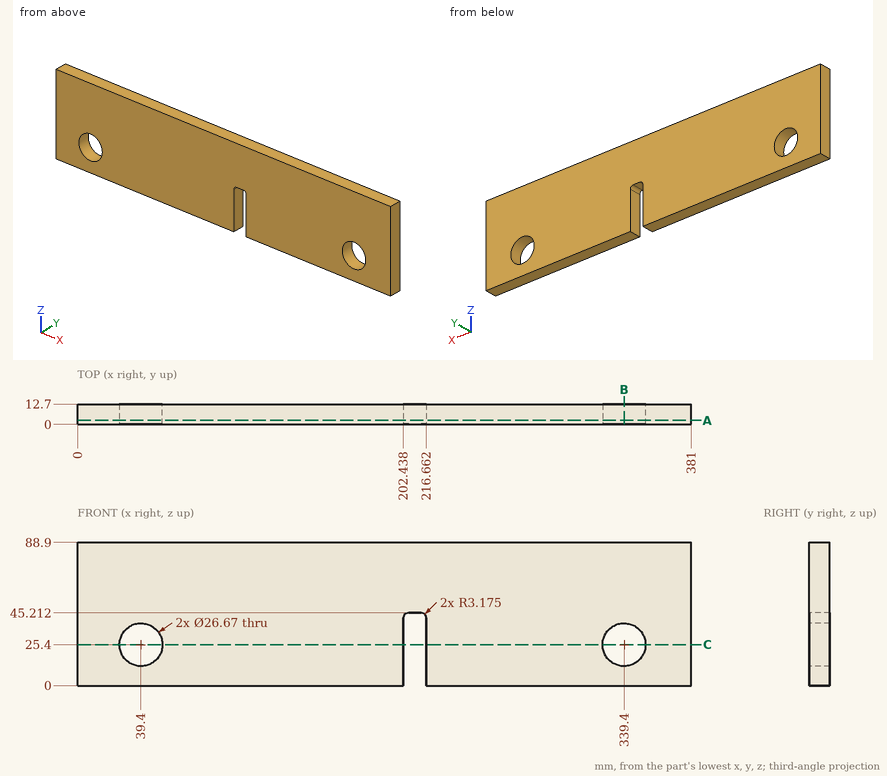
The drawing under review shows one solid part. Ordinate dimensions are in mm from its lowest x, y, z. Round coordinates to 2 decimals unless told otherwise and drop trailing zeros. Loops run counter-clockwise (first coordinate to the right, second up) from the corner with the lowest first, then second, coordinate; pieces in that order, holes last. Notation, with made-up numbers: (13, 89.25) -> (40, 89.25) arc R27 cw to (40, 108.25) -> close; hole circle Ø7 at (22, 71.25). An arc over 180 degrees is marked (long way). One line per question, with ' | ' between items. Start each with the question number.
Item 1: Add section B-B, the plane x = 339.4. Write out the cut boundary in (y, z) (3 decimals), then the cut area to 3 significant figures.
Item 2: Wall thickness on line 1 along Z through (x, y) = (39.4, 6.75) (3 decimals); line 2 along X through (y, z) = (10.5, 25); line 3 along X through (y, z) = (2.75, 28.5): over which ranges is each line inside the solid? List them lowest first. Write a range as [from, to].
Item 3: Add section A-A, the plane y = 2.5. Write out the cut boundary in (x, z) (3 decimals), then the cut area to 3 significant figures.
Item 4: Add section C-C, the plane z = 25.4. Write out the cut boundary in (x, y) (3 decimals), then the cut area to 3 significant figures.
Item 5: For pin 1 (1.5 mm diameter, centred on x = 125.5, y = 2, fed in from -Z), flat-tipped, find the tip position at first contact; note if it passes through.
Return value:
1) outline: (0, 0) -> (12.7, 0) -> (12.7, 12.065) -> (0, 12.065) -> close; (0, 38.735) -> (12.7, 38.735) -> (12.7, 88.9) -> (0, 88.9) -> close | area: 790 mm2
2) line 1: z = [0, 12.065], [38.735, 88.9] | line 2: x = [0, 26.07], [52.73, 202.44], [216.66, 326.07], [352.73, 381] | line 3: x = [0, 26.43], [52.37, 202.44], [216.66, 326.43], [352.37, 381]
3) outline: (0, 0) -> (202.438, 0) -> (202.438, 42.037) arc R3.175 cw to (205.613, 45.212) -> (213.487, 45.212) arc R3.175 cw to (216.662, 42.037) -> (216.662, 0) -> (381, 0) -> (381, 88.9) -> (0, 88.9) -> close; hole circle Ø26.67 at (39.4, 25.4); hole circle Ø26.67 at (339.4, 25.4) | area: 32,100 mm2
4) outline: (0, 0) -> (26.065, 0) -> (26.065, 12.7) -> (0, 12.7) -> close; (52.735, 0) -> (202.438, 0) -> (202.438, 12.7) -> (52.735, 12.7) -> close; (216.662, 0) -> (326.065, 0) -> (326.065, 12.7) -> (216.662, 12.7) -> close; (352.735, 0) -> (381, 0) -> (381, 12.7) -> (352.735, 12.7) -> close | area: 3,980 mm2
5) pin 1: stops at z = 0
